The listing builds one solid part. Answer for the finished solid, in the listing's coordinates (mm). A direction names the side the tool comes from. Give positions to 0.01 mm unless a question says otherwise; leave off trailing zeros. Order: outer loops, then holes, each group sorted by start corner. A loop starts at its lowest first (then second) coordinate and runs counter-clockwise, first axis right, second up. Notation, with made-up numbers: (88.25, 5.5) - (108.25, 5.5) arc R33 cw to (108.25, 35.5) - close; hole circle Ø5 at (-24, -9.75). An arc over 180 degrees is marked (long way). Use CSV: the item, a comma, the result in double quotes.
```python
from build123d import *

# Parameters (mm, degrees)
SKETCH_1_R      = 3.1
EXTRUDE_1_DEPTH = 2


with BuildPart() as part:
    # 草图1 → 凸台-拉伸1 (new body)
    with BuildSketch(Plane(origin=(0, 0, 0), x_dir=(1, 0, 0), z_dir=(0, 1, 0))):
        Polygon((-187.609763817, 175.878092516), (-187.609763817, 235.878092516), (-127.609763817, 235.878092516), (-127.609763817, 295.878092516), (152.390236183, 295.878092516), (152.390236183, 235.878092516), (212.390236183, 235.878092516), (212.390236183, 175.878092516), (272.390236183, 175.878092516), (272.390236183, -204.121907484), (212.390236183, -204.121907484), (212.390236183, -264.121907484), (152.390236183, -264.121907484), (152.390236183, -324.121907484), (-127.609763817, -324.121907484), (-127.609763817, -264.121907484), (-187.609763817, -264.121907484), (-187.609763817, -204.121907484), (-247.609763817, -204.121907484), (-247.609763817, 175.878092516), align=None)
        with Locations(Location((-112.609763817, -279.121907484, 0), (0, 0, 270))):
            Circle(SKETCH_1_R, mode=Mode.SUBTRACT)
        with Locations(Location((-82.609763817, -279.121907484, 0), (0, 0, 270))):
            Circle(SKETCH_1_R, mode=Mode.SUBTRACT)
        with Locations(Location((-112.609763817, -309.121907484, 0), (0, 0, 270))):
            Circle(SKETCH_1_R, mode=Mode.SUBTRACT)
        with Locations(Location((-82.609763817, -309.121907484, 0), (0, 0, 270))):
            Circle(SKETCH_1_R, mode=Mode.SUBTRACT)
        with Locations(Location((-232.609763817, -159.121907484, 0), (0, 0, 270))):
            Circle(SKETCH_1_R, mode=Mode.SUBTRACT)
        with Locations(Location((-202.609763817, -159.121907484, 0), (0, 0, 270))):
            Circle(SKETCH_1_R, mode=Mode.SUBTRACT)
        with Locations(Location((-232.609763817, -189.121907484, 0), (0, 0, 270))):
            Circle(SKETCH_1_R, mode=Mode.SUBTRACT)
        with Locations(Location((-202.609763817, -189.121907484, 0), (0, 0, 270))):
            Circle(SKETCH_1_R, mode=Mode.SUBTRACT)
        with Locations(Location((257.390236183, -189.121907484, 0), (0, 0, 270))):
            Circle(SKETCH_1_R, mode=Mode.SUBTRACT)
        with Locations(Location((227.390236183, -189.121907484, 0), (0, 0, 270))):
            Circle(SKETCH_1_R, mode=Mode.SUBTRACT)
        with Locations(Location((227.390236183, -159.121907484, 0), (0, 0, 270))):
            Circle(SKETCH_1_R, mode=Mode.SUBTRACT)
        with Locations(Location((257.390236183, -159.121907484, 0), (0, 0, 270))):
            Circle(SKETCH_1_R, mode=Mode.SUBTRACT)
        with Locations(Location((227.390236183, 160.878092516, 0), (0, 0, 270))):
            Circle(SKETCH_1_R, mode=Mode.SUBTRACT)
        with Locations(Location((257.390236183, 160.878092516, 0), (0, 0, 270))):
            Circle(SKETCH_1_R, mode=Mode.SUBTRACT)
        with Locations(Location((257.390236183, 130.878092516, 0), (0, 0, 270))):
            Circle(SKETCH_1_R, mode=Mode.SUBTRACT)
        with Locations(Location((227.390236183, 130.878092516, 0), (0, 0, 270))):
            Circle(SKETCH_1_R, mode=Mode.SUBTRACT)
        with Locations(Location((-232.609763817, 160.878092516, 0), (0, 0, 270))):
            Circle(SKETCH_1_R, mode=Mode.SUBTRACT)
        with Locations(Location((-202.609763817, 160.878092516, 0), (0, 0, 270))):
            Circle(SKETCH_1_R, mode=Mode.SUBTRACT)
        with Locations(Location((-202.609763817, 130.878092516, 0), (0, 0, 270))):
            Circle(SKETCH_1_R, mode=Mode.SUBTRACT)
        with Locations(Location((-232.609763817, 130.878092516, 0), (0, 0, 270))):
            Circle(SKETCH_1_R, mode=Mode.SUBTRACT)
        with Locations(Location((-232.609763817, 0.878092516, 0), (0, 0, 270))):
            Circle(SKETCH_1_R, mode=Mode.SUBTRACT)
        with Locations(Location((-202.609763817, 0.878092516, 0), (0, 0, 270))):
            Circle(SKETCH_1_R, mode=Mode.SUBTRACT)
        with Locations(Location((-202.609763817, -29.121907484, 0), (0, 0, 270))):
            Circle(SKETCH_1_R, mode=Mode.SUBTRACT)
        with Locations(Location((-232.609763817, -29.121907484, 0), (0, 0, 270))):
            Circle(SKETCH_1_R, mode=Mode.SUBTRACT)
        with Locations(Location((257.390236183, -29.121907484, 0), (0, 0, 270))):
            Circle(SKETCH_1_R, mode=Mode.SUBTRACT)
        with Locations(Location((227.390236183, -29.121907484, 0), (0, 0, 270))):
            Circle(SKETCH_1_R, mode=Mode.SUBTRACT)
        with Locations(Location((227.390236183, 0.878092516, 0), (0, 0, 270))):
            Circle(SKETCH_1_R, mode=Mode.SUBTRACT)
        with Locations(Location((257.390236183, 0.878092516, 0), (0, 0, 270))):
            Circle(SKETCH_1_R, mode=Mode.SUBTRACT)
        with Locations(Location((137.390236183, -309.121907484, 0), (0, 0, 270))):
            Circle(SKETCH_1_R, mode=Mode.SUBTRACT)
        with Locations(Location((107.390236183, -309.121907484, 0), (0, 0, 270))):
            Circle(SKETCH_1_R, mode=Mode.SUBTRACT)
        with Locations(Location((107.390236183, -279.121907484, 0), (0, 0, 270))):
            Circle(SKETCH_1_R, mode=Mode.SUBTRACT)
        with Locations(Location((137.390236183, -279.121907484, 0), (0, 0, 270))):
            Circle(SKETCH_1_R, mode=Mode.SUBTRACT)
        with Locations(Location((107.390236183, 280.878092516, 0), (0, 0, 270))):
            Circle(SKETCH_1_R, mode=Mode.SUBTRACT)
        with Locations(Location((137.390236183, 280.878092516, 0), (0, 0, 270))):
            Circle(SKETCH_1_R, mode=Mode.SUBTRACT)
        with Locations(Location((137.390236183, 250.878092516, 0), (0, 0, 270))):
            Circle(SKETCH_1_R, mode=Mode.SUBTRACT)
        with Locations(Location((107.390236183, 250.878092516, 0), (0, 0, 270))):
            Circle(SKETCH_1_R, mode=Mode.SUBTRACT)
        with Locations(Location((-112.609763817, 280.878092516, 0), (0, 0, 270))):
            Circle(SKETCH_1_R, mode=Mode.SUBTRACT)
        with Locations(Location((-82.609763817, 280.878092516, 0), (0, 0, 270))):
            Circle(SKETCH_1_R, mode=Mode.SUBTRACT)
        with Locations(Location((-82.609763817, 250.878092516, 0), (0, 0, 270))):
            Circle(SKETCH_1_R, mode=Mode.SUBTRACT)
        with Locations(Location((-112.609763817, 250.878092516, 0), (0, 0, 270))):
            Circle(SKETCH_1_R, mode=Mode.SUBTRACT)
        with BuildLine():
            Line((-37.609763817, 150.878092516), (62.390236183, 150.878092516))
            ThreePointArc((62.390236183, 150.878092516), (112.390236183, 100.878092516), (62.390236183, 50.878092516))
            Line((62.390236183, 50.878092516), (-37.609763817, 50.878092516))
            ThreePointArc((-37.609763817, 50.878092516), (-87.609763817, 100.878092516), (-37.609763817, 150.878092516))
        make_face(mode=Mode.SUBTRACT)
        with BuildLine():
            Line((-37.609763817, -179.121907484), (62.390236183, -179.121907484))
            ThreePointArc((62.390236183, -179.121907484), (112.390236183, -129.121907484), (62.390236183, -79.121907484))
            Line((62.390236183, -79.121907484), (-37.609763817, -79.121907484))
            ThreePointArc((-37.609763817, -79.121907484), (-87.609763817, -129.121907484), (-37.609763817, -179.121907484))
        make_face(mode=Mode.SUBTRACT)
    extrude(amount=EXTRUDE_1_DEPTH)


solid = part.part
```
Item 1: Which of the six approach directions +Z, -Z, +X, -X, +Y, -Y give full straight-line access (tool end or side, diameter ignored) to faces 1 (the face through (16, 2, 10)), 2 (the face through (112.38, 0.99, -101.98))?
Taken from the geometry:
face 1,"+Z, -Z, +X, -X, +Y"
face 2,"+Y, -Y"
Item 2: The mould has two halves that part along X. Classify faces 3 (the face through (16, 0, 10)), 4 (the face through (-87.598, 0.986, 128.022)): +X half, -X half, draft (parallel to the pull), parting line (faces both ways), or undercut.
Taken from the geometry:
face 3,"draft"
face 4,"undercut"
Item 3: Each of these flat-tipped pins is pushed along its axis until it touches: pin 1 (3.5 mm diameter, centred on x = 107.39, z = -250.88, fed in from -Y); pin 2 (0.6 mm diameter, centred on y = 1.5, z = -272, fed in from -X); pin 3 (0.6 mm diameter, centred on x = -221.5, y = 1.5, fed in from -Z). Where does it stop, or does it pass through?
Taken from the geometry:
pin 1,"through"
pin 2,"x = -127.61"
pin 3,"z = -175.88"
Item 4: The part is cut by section B-B (z = -143.5). Give the vertices of the cut face in (x, y).
Taken from the geometry:
outline,"(-247.61, 0) - (-63.75, 0) - (-63.75, 2) - (-247.61, 2) - close; (88.53, 0) - (272.39, 0) - (272.39, 2) - (88.53, 2) - close"
Item 5: The part is cut by section A-A (x = -70.5). Give the vertices of the cut face in (y, z), and give its area (3 significant figures).
Taken from the geometry:
outline,"(0, -295.88) - (2, -295.88) - (2, -138.54) - (0, -138.54) - close; (0, -63.22) - (2, -63.22) - (2, 91.46) - (0, 91.46) - close; (0, 166.78) - (2, 166.78) - (2, 324.12) - (0, 324.12) - close"
area,"939 mm^2"
Item 6: The part is cut by section D-D (z = 254.5). Give the vertices of the cut face in (x, y).
Taken from the geometry:
outline,"(-187.61, 0) - (212.39, 0) - (212.39, 2) - (-187.61, 2) - close"
Item 7: The part is cut by section C-C (x = 74.5). Give the vertices of the cut face in (y, z), and give its area (3 significant figures).
Taken from the geometry:
outline,"(0, -295.88) - (2, -295.88) - (2, -149.39) - (0, -149.39) - close; (0, -52.37) - (2, -52.37) - (2, 80.61) - (0, 80.61) - close; (0, 177.63) - (2, 177.63) - (2, 324.12) - (0, 324.12) - close"
area,"852 mm^2"
Item 8: Find the intervals of material crossed by line 1 along Z through (x, y) = (59, 0.7); line 2 along Z through (x, y) = (78, 1); line 3 along Z through (x, y) = (-214, 0.85), in increasing order.
Taken from the geometry:
line 1,"-295.88 to -150.88, -50.88 to 79.12, 179.12 to 324.12"
line 2,"-295.88 to -148.38, -53.38 to 81.62, 176.62 to 324.12"
line 3,"-175.88 to 204.12"
